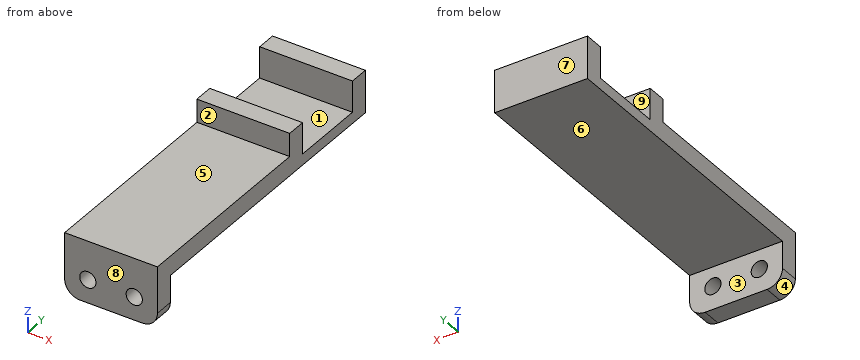
```python
from build123d import *

# Parameters (mm, degrees)
SKETCH1_W           = 12
SKETCH1_H           = 8
BOSS_EXTRUDE1_DEPTH = 2.5
FILLET1_R           = 2
SKETCH2_R           = 1.05
CUT_EXTRUDE1_DEPTH  = 2.5
SKETCH3_W           = 12
SKETCH3_H           = 2.5
BOSS_EXTRUDE2_DEPTH = 37.9
SKETCH5_W           = 12
SKETCH5_H           = 2.5
BOSS_EXTRUDE4_DEPTH = 3
SKETCH6_W           = 12
SKETCH6_H           = 2.5
BOSS_EXTRUDE5_DEPTH = 3
SKETCH7_W           = 1.05
SKETCH7_H           = 9.7
CUT_EXTRUDE2_DEPTH  = 15


with BuildPart() as part:
    # Sketch1 → Boss-Extrude1 (new body)
    with BuildSketch(Plane(origin=(0, 0, 0), x_dir=(1, 0, 0), z_dir=(0, 1, 0))):
        Rectangle(SKETCH1_W, SKETCH1_H)
    extrude(amount=BOSS_EXTRUDE1_DEPTH)

    # Fillet1
    fillet1_edges = [part.edges().sort_by_distance(p)[0] for p in [
        (-6, 1.25, -4),
        (6, 1.25, -4),
    ]]
    fillet(fillet1_edges, radius=FILLET1_R)

    # Sketch2 → Cut-Extrude1 (cut)
    with BuildSketch(Plane(origin=(0, 2.5, 0), x_dir=(1, 0, 0), z_dir=(0, 1, 0))):
        with Locations(Location((3, 1, 0), (0, 0, 270))):
            Circle(SKETCH2_R)
        with Locations(Location((-3, 1, 0), (0, 0, 270))):
            Circle(SKETCH2_R)
    extrude(amount=-CUT_EXTRUDE1_DEPTH, mode=Mode.SUBTRACT)

    # Sketch3 → Boss-Extrude2 (add)
    with BuildSketch(Plane(origin=(0, 2.5, 0), x_dir=(1, 0, 0), z_dir=(0, 1, 0))):
        with Locations((0, -2.75)):
            Rectangle(SKETCH3_W, SKETCH3_H)
    extrude(amount=BOSS_EXTRUDE2_DEPTH)

    # Sketch5 → Boss-Extrude4 (add)
    with BuildSketch(Plane.XY.offset(4)):
        with Locations((0, 39.15)):
            Rectangle(SKETCH5_W, SKETCH5_H)
    extrude(amount=BOSS_EXTRUDE4_DEPTH)

    # Sketch6 → Boss-Extrude5 (add)
    with BuildSketch(Plane.XY.offset(4)):
        with Locations((0, 26.95)):
            Rectangle(SKETCH6_W, SKETCH6_H)
    extrude(amount=BOSS_EXTRUDE5_DEPTH)

    # Sketch7 → Cut-Extrude2 (cut)
    with BuildSketch(Plane.ZY.offset(6)):
        with Locations((3.475, 33.05)):
            Rectangle(SKETCH7_W, SKETCH7_H)
    extrude(amount=-CUT_EXTRUDE2_DEPTH, mode=Mode.SUBTRACT)


solid = part.part
```
The listing builds one solid part. Answer for the finished solid, in the listing's coordinates (mm). Face numbers are marked on the shaded views. A direction names the side the tool comes from. Coordinates: 2 decimals unless noted, no trailing zeros. Write each loop counter-clockwise with the first axis right and the second up, starting at its lowest first coordinate (ties: lowest second). Pieces come first, ordered by that corner, then holes. Notation, with made-up numbers: (86, 88.25) - (94, 88.25) arc R26 cw to (94, 112.25) - close; hole circle Ø1 at (65, 78). An arc over 180 degrees is marked (long way). Return JSON: item names as keys, results as strings. Group by question number.
Q1. For a pull along Y with two mould halves and no side action, classify the marked faces 1, 2, 3 and 4 as +Y half, -Y half, draft (parallel to the pull), parting line (faces both ways), or undercut.
Q2. The part is cut by section A-A on z = -1. Write down the section's boundary in (x, y), and give its area (3 significant figures).
Q3. Flat-ended cylindrical pins translate along their axes: pin 1 Ø3.5 at (x, z) = (-3, -1) entering from +Y; pin 2 Ø6 at (x, y) = (1, 10) entering from -Z; pin 3 Ø3 at (x, y) = (0.5, 32) entering from +Z. Find the tip coordinate at first contact, or state that the pin passes through.
Q4. Which of the six approach directions +Z, -Z, +X, -X, +Y, -Y give full straight-line access (tool end or side, diameter ignored) to the marked faces 5, 6, 7, 8 and 9?
Q5. The part is cut by section D-D on y = 14. Write down the section's boundary in (x, z), and give its area (3 significant figures).
Q6. The part is cut by section C-C on x = 0. Write down the section's boundary in (y, z), and give its area (3 significant figures).
Q7. The part is cut by section B-B on x = 3. Write down the section's boundary in (y, z).
Q8. Find the intervals of material crossed by line 1 along X through (y, z) = (1.15, -1); line 2 along Y through (x, z) = (5.25, 6.75); line 3 along Y through (x, z) = (5, 3.25), in increasing order. Write a range as [from, to].
Evaluation:
{
 "1": {"face 1": "undercut", "face 2": "-Y half", "face 3": "+Y half", "face 4": "draft"},
 "2": {"outline": "(-6, 0) - (-4.05, 0) - (-4.05, 2.5) - (-6, 2.5) - close; (-1.95, 0) - (1.95, 0) - (1.95, 2.5) - (-1.95, 2.5) - close; (4.05, 0) - (6, 0) - (6, 2.5) - (4.05, 2.5) - close", "area": "19.5 mm2"},
 "3": {"pin 1": "stops at y = 2.5", "pin 2": "stops at z = 1.5", "pin 3": "stops at z = 2.95"},
 "4": {"face 5": "+Z, +X, -X, -Y", "face 6": "-Z, +X, -X, +Y", "face 7": "+Z, -Z, +X, -X, +Y", "face 8": "+Z, -Z, +X, -X, -Y", "face 9": "+Z, +X, -X"},
 "5": {"outline": "(-6, 1.5) - (6, 1.5) - (6, 4) - (-6, 4) - close", "area": "30.0 mm2"},
 "6": {"outline": "(0, -4) - (2.5, -4) - (2.5, 1.5) - (40.4, 1.5) - (40.4, 7) - (37.9, 7) - (37.9, 2.95) - (28.2, 2.95) - (28.2, 7) - (25.7, 7) - (25.7, 4) - (0, 4) - close", "area": "120 mm2"},
 "7": {"outline": "(0, -4) - (2.5, -4) - (2.5, -2.05) - (0, -2.05) - close; (0, 0.05) - (2.5, 0.05) - (2.5, 1.5) - (40.4, 1.5) - (40.4, 7) - (37.9, 7) - (37.9, 2.95) - (28.2, 2.95) - (28.2, 7) - (25.7, 7) - (25.7, 4) - (0, 4) - close"},
 "8": {"line 1": "x = [-6, -4.05], [-1.95, 1.95], [4.05, 6]", "line 2": "y = [25.7, 28.2], [37.9, 40.4]", "line 3": "y = [0, 28.2], [37.9, 40.4]"}
}
